Geometry: see drawing. Coordinates: mm, zero at the bounding-box minimum. A direction names the side the tool comes from. Round coordinates to 2 decimals unless told otherwise and drop trailing zeros. Write each loop counter-clockwise with the first axis right and the second up, starting at its lowest first coordinate (ties: lowest second). Pieces come first, ordered by that corner, then holes. Notation, with made-up numbers: (-23, 12.25) - (12, 12.25) arc R22 cw to (12, 29.25) - close; hole circle Ø5 at (-16.75, -16). An arc over 180 degrees is marked (long way). One line per item, written item: value. Start each with the question number.
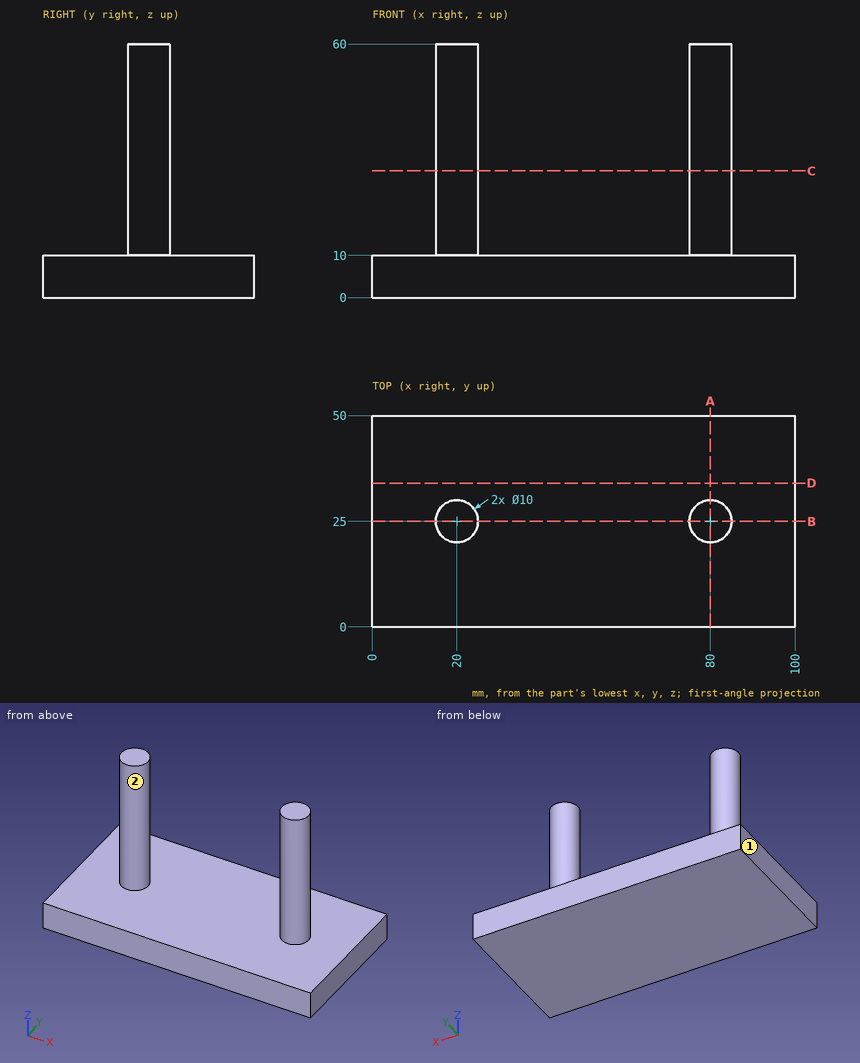
Q1. Cut plane B-B, the plane y = 25. Output: boundary loops of the cut face in (x, z).
Q2. Cut plane A-A, the plane x = 80. Output: boundary loops of the cut face in (y, z), and give its area (3 significant figures).
Q3. Material intervals for probe 1 along X at (y, z) = (25.5, 24.5); probe 2 along Z at (x, y) = (33.5, 7); probe 3 along X at (y, z) = (28, 26), sorted ascending. Write a range as from..to.
Q4. Cut plane C-C, the plane z = 30. Output: boundary loops of the cut face in (x, y), and give its area (3 significant figures).
Q5. Access query for the marked faces 1 and 2. Directions: +Z, -Z, +X, -X, +Y, -Y. A direction counts if a zero-diameter tool reaches every point of the face in a straight line with its end or side. Return the directions, or none.
Q6. Cut plane D-D, the plane y = 34. Output: boundary loops of the cut face in (x, z).
Q7. Contact query for flat-ended pins moving along their axis: pin 1 Ø15 at (x, y) = (54, 25) entering from +Z; pin 2 Ø1 at (x, y) = (60, 39) entering from -Z; pin 3 Ø1 at (x, z) = (76, 41.5) entering from -Y; pin 4 Ø4 at (x, z) = (78, 17.5) entering from +Y. Output: stop coordinate, or through.
A:
1. outline: (0, 0) - (100, 0) - (100, 10) - (85, 10) - (85, 60) - (75, 60) - (75, 10) - (25, 10) - (25, 60) - (15, 60) - (15, 10) - (0, 10) - close
2. outline: (0, 0) - (50, 0) - (50, 10) - (30, 10) - (30, 60) - (20, 60) - (20, 10) - (0, 10) - close
2. area: 1,000 mm²
3. probe 1: x = 15.03..24.97, 75.03..84.97
3. probe 2: z = 0..10
3. probe 3: x = 16..24, 76..84
4. outline: circle Ø10 at (20, 25); circle Ø10 at (80, 25)
4. area: 157 mm²
5. face 1: +Z, -Z, -X, +Y, -Y
5. face 2: +Z
6. outline: (0, 0) - (100, 0) - (100, 10) - (0, 10) - close
7. pin 1: stops at z = 10
7. pin 2: stops at z = 0
7. pin 3: stops at y = 21.43
7. pin 4: stops at y = 30
